Here's how the part is built. I have some questions about the finished solid (model axes, mm). A direction names the side the tool comes from. Give positions to 0.01 mm unless a question says otherwise; leave off trailing zeros. Loops run counter-clockwise (first coordinate to the right, second up) from the corner with the lowest first, then second, coordinate; pieces in that order, holes last. Notation, with made-up numbers: (-14, 25.25) - (5, 25.25) arc R19 cw to (5, 46.25) - close; hole circle Ø8 at (-27, 64.5). An arc over 180 degrees is marked (long way). Use one line per item in the form item = value.
Autodesk Inventor part; units mm, degrees
ref_plane "Plano de trabajo1" through (31.12, -8, -69) normal (-1, 0, 0) x (0, 0, 1)
ref_plane "Plano de trabajo2" through (33.12, -8, -69) normal (-1, 0, 0) x (0, 0, 1)
ref_plane "Plano de trabajo4" through (31.12, -8, -72) normal (-1, 0, 0) x (0, 0, 1)
sketch "Boceto2" plane through (0, 0, 0) normal (1, 0, 0) x (0, 1, 0)
  line L0 (0, 0) -> (-67, 0)
  line L1 (-67, 0) -> (-67, 6)
  line L2 (-67, 6) -> (0, 6)
  line L3 (0, 6) -> (0, 0)
  dimension "d2" = 67
  dimension "d3" = 6
extrude "Extrusión2" add sketch "Boceto2" along normal blind 65
sketch "Boceto3" plane through (65, 0, 0) normal (1, 0, 0) x (0, 0, -1)
  line L0 (-6, -5) -> (72, -5)
  line L1 (-6, -8) -> (-6, -5)
  line L2 (72, -8) -> (-6, -8)
  line L3 (72, -5) -> (72, -8)
  line L4 (-6, 0) -> (-6, -67)
  line L5 (-6, -67) -> (0, -67)
  line L6 (0, -67) -> (0, 0)
  line L7 (0, 0) -> (-6, 0)
  point P0 (0, -5)
ref_plane "Plano de trabajo1" through (31.12, -8, -69) normal (-1, 0, 0) x (0, 0, 1)
ref_plane "Plano de trabajo2" through (33.12, -8, -69) normal (-1, 0, 0) x (0, 0, 1)
ref_plane "Plano de trabajo4" through (31.12, -8, -72) normal (-1, 0, 0) x (0, 0, 1)
extrude "Extrusión3" cut sketch "Boceto3" against normal up to surface (33.88 mm away) contours L0 L6 L2 L1 | L2 L6 L5 L4
sketch "Boceto4" plane through (0, 0, 6) normal (0, 1, 0) x (1, 0, 0)
  circle A0 centre (34.12, 75) radius 1.5
  circle A1 centre (62, 75) radius 1.5
  line L0 (65, 0) -> (65, 78)
  line L1 (65, 78) -> (31.12, 78)
  line L2 (65, 0) -> (31.12, 0)
  line L3 (0, 6) -> (0, 0)
  line L4 (0, 0) -> (65, 0)
  line L5 (65, 6) -> (65, 0)
  line L6 (0, 6) -> (65, 6)
  line L7 (0, 0) -> (65, 0)
  line L8 (65, 0) -> (62, 0)
  line L9 (65, 0) -> (68, 0) construction
  line L10 (62, 0) -> (62, 3)
  circle A2 centre (62, 3) radius 2.1
  circle A3 centre (36.12, 3) radius 2.1
  circle A4 centre (36.12, 3) radius 1.5
  circle A5 centre (62, 3) radius 1.5
  line L11 (31.12, 0) -> (31.12, 78)
  point P0 (33.12, 0)
  dimension "d8" = 3
  dimension "d9" = 180
  dimension "d10" = 3
  dimension "d11" = 4.2
  dimension "d12" = 4.2
hole "Agujero1" at (36.12, 0, 3) at (62, 0, 3) direction (0, -1, 0) diameter 4.2 depth 5
sketch "Boceto5" plane through (0, -67, 6) normal (0, 0, 1) x (1, 0, 0)
  circle A0 centre (5, 57) radius 2.1
  circle A1 centre (5, 5) radius 2.1
  point P0 (0, 67)
hole "Agujero2" at (5, -10, 6) at (5, -62, 6) direction (0, 0, -1) diameter 3.2 depth 5
sketch "Boceto6" plane through (31.12, -67, 6) normal (1, 0, 0) x (0, 0, -1)
  line L0 (6, 62) -> (0, 62)
  line L1 (0, 0) -> (0, 62)
  line L2 (6, 0) -> (0, 0)
  line L3 (6, 62) -> (6, 0)
  line L4 (6, 0) -> (3, 0)
  line L5 (3, 0) -> (3, 62)
  line L6 (3, 62) -> (6, 62)
  line L7 (6, 62) -> (6, 0)
  point P0 (6, 67)
  point P1 (3, 0)
ref_plane "Plano de trabajo3" through (10, -67, -66) normal (1, 0, 0) x (0, 1, 0)
extrude "Extrusión4" cut sketch "Boceto6" against normal up to surface (21.12 mm away) contours L3 L2 L5 L0
sketch "Boceto7" plane through (31.12, -67, 6) normal (1, 0, 0) x (0, 0, -1)
  line L0 (3, 0) -> (3, 62)
  line L1 (3, 62) -> (0, 62)
  line L2 (0, 0) -> (0, 62)
  line L3 (3, 0) -> (0, 0)
  line L4 (0, 62) -> (78, 62)
  line L5 (0, 59) -> (0, 62)
  line L6 (78, 59) -> (0, 59)
  line L7 (78, 62) -> (78, 59)
  point P0 (6, 67)
  point P1 (3, 59)
extrude "Extrusión5" add sketch "Boceto7" along normal blind 6 contours L3 L2 L6 L0
properties part number "Lateral derecho"
(1) If we section it at B-B (x = 5): List the corners of the cut face in (y, z) for me, plus the area to 3 significant figures.
Geometry says:
outline = (-67, 0) - (0, 0) - (0, 6) - (-8.4, 6) - (-8.4, 1) - (-11.6, 1) - (-11.6, 6) - (-60.4, 6) - (-60.4, 1) - (-63.6, 1) - (-63.6, 6) - (-67, 6) - close
area = 370 mm²
(2) If we section it at D-D (x = 18): List the corners of the cut face in (y, z) for me.
Geometry says:
outline = (-67, 3) - (-5, 3) - (-5, 0) - (0, 0) - (0, 6) - (-67, 6) - close
(3) If we section it at A-A (y = -62): List the corners of the cut face in (x, z) for me, plus the area to 3 significant figures.
Geometry says:
outline = (0, 0) - (10, 0) - (10, 3) - (37.12, 3) - (37.12, 6) - (6.6, 6) - (6.6, 1) - (3.4, 1) - (3.4, 6) - (0, 6) - close
area = 125 mm²
(4) For faces 4 (the flat face through (31.12, -6, 5)), 5 (the flat face through (37.12, -37, 5)), 6 (the flat face through (10, -36, 2)), 7 (the flat face through (5, -62, 1)), which set-ups out of +Z, -Z, +X, -X, +Y, -Y let a thin tool reach every point of the face, with its end or its side?
Geometry says:
face_4 = +Z, -Z, +X
face_5 = +Z, -Z, +X, -Y
face_6 = -Z, +X, -Y
face_7 = +Z
(5) If we section it at C-C (y = -52): List the corners of the cut face in (x, z) for me, plus the area to 3 significant figures.
Geometry says:
outline = (0, 0) - (10, 0) - (10, 3) - (37.12, 3) - (37.12, 6) - (0, 6) - close
area = 141 mm²
(6) If I drill on probe 1 along X at (y, z) = (-1.35, 3); probe 2 along Y at (x, z) = (5, 2.15); probe 3 along X at (y, z) = (-10, 4), over which ranges is the centre line in solid material (lowest first)?
Geometry says:
probe_1 = 0 to 34.02, 38.22 to 59.9, 64.1 to 65
probe_2 = -67 to -63.6, -60.4 to -11.6, -8.4 to 0
probe_3 = 0 to 3.4, 6.6 to 37.12
(7) For P1, Ø2.5, axis at y = -26.5, z = 5, coming from the +X side; P2, Ø0.9, axis at x = 35, z = 4, coming from the +Y side; P3, Ø1.5, axis at y = -40.5, z = 1, coming from the +X side, each with a flat end and sliding along its axis, tell me the tip position at first contact or that it passes through.
Geometry says:
P1 = 37.12
P2 = -8
P3 = 10
(8) Thinking about a two-plate mould opening in Y: for faces 1 (the flat face through (5, -10, 1)), 2 (the flat face through (32, 0, 3)), 3 (the flat face through (0, -34, 3)), which applies, pulls with the +Y half, pulls with the -Y half, needs draft (parallel to the pull), parting line crosses it, or undercut?
Geometry says:
face_1 = undercut
face_2 = pulls with the +Y half
face_3 = needs draft
